```python
from build123d import *

# Parameters (mm, degrees)
FILLET1_R           = 0.25
SKETCH2_W           = 20.2
SKETCH2_H           = 0.75
SKETCH3_R           = 1.2125
BOSS_EXTRUDE1_DEPTH = 10
SKETCH4_R           = 1.5
CUT_EXTRUDE1_DEPTH  = 15
SKETCH6_R           = 5
BOSS_EXTRUDE2_DEPTH = 1.5


with BuildPart() as part:
    # Sketch1 → Revolve1 (revolve)
    with BuildSketch(Plane.XY):
        Polygon((16.42, 1.5875), (20.555933238, 0.375), (20.555933238, -0.375), (16.42, -1.5875), (-16.42, -1.5875), (-16.42, 1.5875), (-15.12, 1.5875), (-15.12, 1.2875), (-14.67, 1.2875), (-14.67, 1.5875), align=None)
    revolve(axis=Axis((-16.42, -1.5875, 0), (1, 0, 0)))

    # Fillet1
    fillet1_edges = [part.edges().sort_by_distance(p)[0] for p in [
        (-16.42, -4.7625, 0),
    ]]
    fillet(fillet1_edges, radius=FILLET1_R)



with BuildPart() as body_2:
    # Sketch2 → Revolve2 (revolve)
    with BuildSketch(Plane.XY):
        with Locations((30.655933238, -1.2125)):
            Rectangle(SKETCH2_W, SKETCH2_H)
    revolve(axis=Axis((20.555933238, -1.5875, 0), (1, 0, 0)))


with BuildPart() as part_1:
    add(part.part)

    add(body_2.part)  # Boss-Extrude1 merges body 2
    # Sketch3 → Boss-Extrude1 (add)
    with BuildSketch(Plane(origin=(20.555933238, 0, 0), x_dir=(0, 0, -1), z_dir=(1, 0, 0))):
        with Locations((0, -1.5875)):
            Circle(SKETCH3_R)
    extrude(amount=-BOSS_EXTRUDE1_DEPTH)

    # Sketch4 → Cut-Extrude1 (cut)
    with BuildSketch(Plane.ZY.offset(16.42)):
        with Locations((0, -1.5875)):
            Circle(SKETCH4_R)
    extrude(amount=-CUT_EXTRUDE1_DEPTH, mode=Mode.SUBTRACT)

    # Sketch6 → Boss-Extrude2 (add)
    with BuildSketch(Plane.ZY.offset(16.42)):
        with Locations((0, -1.5875)):
            Circle(SKETCH6_R)
    extrude(amount=BOSS_EXTRUDE2_DEPTH)


solid = part_1.part
```
Read the model definition and answer for the solid it produces. Units are mm, in the model's axes. A direction names the side the tool comes from. Round coordinates to 2 decimals unless told otherwise and drop trailing zeros. Write each loop counter-clockwise with the first axis right and the second up, starting at its lowest first coordinate (ties: lowest second). Pieces come first, ordered by that corner, then holes. Notation, with made-up numbers: (-33.75, 49.5) -> (18.25, 49.5) arc R16 ccw to (18.25, 79.5) -> close; hole circle Ø6 at (-25, -4). An arc over 180 degrees is marked (long way). Answer in a Markdown table with one row per item. Add a question column.
1) Determine the mould class of faces 4 (the face through (-17.92, -2, 0)), 5 (the face through (30.797, -2.337, 0.033)), 6 (the face through (-1.42, -2, 0)) for opening direction Z: pulls with the +Z half, pulls with the -Z half, needs draft (parallel to the pull), parting line crosses it, or undercut.
2) Given P1, Ø6, axis at x = 18, z = -3.5, coming from the +Y side; P2, Ø1.5, axis at x = -1, z = -3.5, coming from the +Y side; P3, Ø2, axis at x = -5.5, z = 1, coming from the +Y side, each flat-ended and moving along its own axis, determine where each tip first touches the part or whether it passes through.
3) Consider line 1 (X direction, y = -0.5, z = 1); line 2 (X direction, y = -3.5, z = -3.5); line 3 (Z direction, x = -3.5, y = -1). Determine where each line is inside the solid, lowest interval first.
4) Which of the six approach directions +Z, -Z, +X, -X, +Y, -Y give full straight-line access (tool end or side, diameter ignored) to faces 1 (the face through (-15.64, 1.44, 0.95)), 2 (the face through (-14.892, -0.042, 2.424)), 3 (the face through (40.756, -2, 0))?
5) Find section D-D, the plane y = 2.25. Determine the outline of the cut face in (x, z), and give its area (3 significant figures).
Findings below:
| question | item | result |
|---|---|---|
| 1 | face 4 | needs draft |
| 1 | face 5 | parting line crosses it |
| 1 | face 6 | undercut |
| 2 | P1 | y = 1.44 |
| 2 | P2 | y = 0 |
| 2 | P3 | y = 1.59 |
| 3 | line 1 | -17.92 to -16.42, -1.42 to 20.56 |
| 3 | line 2 | -17.92 to -16.42 |
| 3 | line 3 | -3.12 to -1.38, 1.38 to 3.12 |
| 4 | face 1 | +X |
| 4 | face 2 | none |
| 4 | face 3 | +Z, -Z, +X, +Y, -Y |
| 5 | outline | (-17.92, -3.21) -> (-16.42, -3.21) -> (-16.42, 3.21) -> (-17.92, 3.21) -> close |
| 5 | area | 9.62 mm² |
